```python
from build123d import *

# Parameters (mm, degrees)
F0_W     = 200
F0_H     = 200
F1_DEPTH = 110
F2_W     = 100
F2_H     = 76.8
F2_H_2   = 113.2
F3_DEPTH = 200
F4_W     = 10
F4_H     = 70
F5_DEPTH = 100
F7_DEPTH = 200
F8_R     = 4.25
F9_DEPTH = 10
F10_R    = 2


with BuildPart() as f1:
    # F0 (on Front) → F1 (new body)
    with BuildSketch(Plane.XZ):
        Rectangle(F0_W, F0_H)
    extrude(amount=F1_DEPTH)

    # F2 (on face) → F3 (cut)
    with BuildSketch(Plane.YZ.offset(100)):
        with Locations((-50, 61.6)):
            Rectangle(F2_W, F2_H)
        with Locations((-50, -43.4)):
            Rectangle(F2_W, F2_H_2)
    extrude(amount=-F3_DEPTH, mode=Mode.SUBTRACT)

    # F4 (on face) → F5 (join)
    with BuildSketch(Plane(origin=(0, -100, 0), x_dir=(-1, 0, 0), z_dir=(0, 1, 0))):
        with Locations((0, -21.8)):
            Rectangle(F4_W, F4_H)
    extrude(amount=F5_DEPTH)

    # F6 (on face) → F7 (cut)
    with BuildSketch(Plane.YZ.offset(5)):
        Polygon((0, 13.2), (-30, 13.2), (-100, -56.8), (0, -56.8), align=None)
    extrude(amount=-F7_DEPTH, mode=Mode.SUBTRACT)

    # F8 (on face) → F9 (cut)
    with BuildSketch(Plane(origin=(0, -100, 0), x_dir=(-1, 0, 0), z_dir=(0, 1, 0))):
        with Locations((-85, 85)):
            Circle(F8_R)
        with Locations((85, 85)):
            Circle(F8_R)
        with Locations((85, -85)):
            Circle(F8_R)
        with Locations((-85, -85)):
            Circle(F8_R)
    extrude(amount=-F9_DEPTH, mode=Mode.SUBTRACT)

    # F10
    f10_edges = [f1.edges().sort_by_distance(p)[0] for p in [
        (0, -100, 23.2),
        (52.5, -100, 13.2),
        (5, -100, -21.8),
        (5, -65, 13.2),
        (0, -30, 13.2),
        (0, -100, -56.8),
        (-5, -65, 13.2),
        (-5, -100, -21.8),
        (-52.5, -100, 13.2),
    ]]
    fillet(f10_edges, radius=F10_R)


solid = f1.part
```
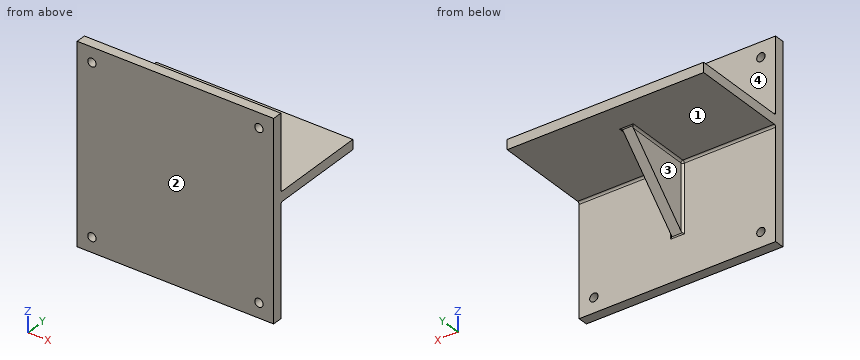
Verification items for the finished model (mm, model axes). Face numbers are marked on the shaded views. A direction names the side the tool comes from. Round coordinates to 2 decimals unless told otherwise and drop trailing zeros. Order: outer loops, then holes, each group sorted by start corner. A loop starts at its lowest first (then second) coordinate and runs counter-clockwise, first axis right, second up.
1) Cross-section at A-A, the plane x = 85. Record the cut outline in (y, z).
Geometry says:
outline: (-110, -100) - (-100, -100) - (-100, -89.25) - (-110, -89.25) - close; (-110, -80.75) - (-100, -80.75) - (-100, 11.2) arc R2 cw to (-98, 13.2) - (0, 13.2) - (0, 23.2) - (-98, 23.2) arc R2 cw to (-100, 25.2) - (-100, 80.75) - (-110, 80.75) - close; (-110, 89.25) - (-100, 89.25) - (-100, 100) - (-110, 100) - close
2) Cross-section at D-D, the plane x = -43. Record the cut outline in (y, z), plus the area to 3 significant figures.
Geometry says:
outline: (-110, -100) - (-100, -100) - (-100, 11.2) arc R2 cw to (-98, 13.2) - (0, 13.2) - (0, 23.2) - (-98, 23.2) arc R2 cw to (-100, 25.2) - (-100, 100) - (-110, 100) - close
area: 3,000 mm2
3) Tool access check on the marked faces 1, 2, 3 and 4. Record the directions out of +Z, -Z, +X, -X, +Y, -Y that give a thin tool (end or side, any length) a straight path to the whole face; none if there is none.
Geometry says:
face 1: -Z, +Y
face 2: +Z, -Z, +X, -X, -Y
face 3: -Z, -X, +Y
face 4: +Z, +X, -X, +Y
4) Depth check by flat-ended pin: pin 1 (3 mm diameter, centred on x = 80, z = 31, fed in from +Y); pin 2 (1 mm diameter, centred on x = -76.5, y = -23.5, fed in from +Z); pin 3 (8 mm diameter, centred on x = 9.5, y = -26.5, fed in from -Z). Enter the tip coordinate at first touch or a pass-through.
Geometry says:
pin 1: stops at y = -100
pin 2: stops at z = 23.2
pin 3: stops at z = 13.19
5) Material ranges on line 1 (Z direction, x = -85, y = -103.25); line 2 (Y direction, x = -71, z = 70.5); line 3 (Z direction, x = 39.5, y = -8), recorded low to high.
Geometry says:
line 1: z = -100 to -89.25, -80.75 to 80.75, 89.25 to 100
line 2: y = -110 to -100
line 3: z = 13.2 to 23.2
6) Cross-section at C-C, the plane y = -51. Record the cut outline in (x, z).
Geometry says:
outline: (-100, 13.2) - (-7, 13.2) arc R2 cw to (-5, 11.2) - (-5, -7.8) - (5, -7.8) - (5, 11.2) arc R2 cw to (7, 13.2) - (100, 13.2) - (100, 23.2) - (-100, 23.2) - close
7) Cross-section at B-B, the plane z = -85. Record the cut outline in (x, y).
Geometry says:
outline: (-100, -110) - (-89.25, -110) - (-89.25, -100) - (-100, -100) - close; (-80.75, -110) - (80.75, -110) - (80.75, -100) - (-80.75, -100) - close; (89.25, -110) - (100, -110) - (100, -100) - (89.25, -100) - close
